Verification items for the finished model (mm, model axes). A direction names the side the tool comes from. Coordinates: 2 decimals unless noted, no trailing zeros. Loops run counter-clockwise (first coordinate to the right, second up) from the corner with the lowest first, then second, coordinate; pieces in that order, holes last. Notation, with made-up numbers: (60, 28.25) -> (93, 28.25) arc R12 cw to (93, 47.25) -> close; hole circle Ø2 at (2.25, 42). An arc over 180 degrees is marked (long way). Write item = value, one per line.
Autodesk Inventor part; units mm, degrees
ref_plane "YZ Plane" through (0, 0, 0) normal (1, 0, 0) x (0, 1, 0)
ref_plane "XZ Plane" through (0, 0, 0) normal (0, 1, 0) x (-1, 0, 0)
ref_plane "XY Plane" through (0, 0, 0) normal (0, 0, 1) x (1, 0, 0)
sketch "Szkic1" plane through (0, 0, 0) normal (0, 0, 1) x (1, 0, 0)
  line L0 (0, 0) -> (17, 0)
  line L1 (17, 0) -> (17, -2)
  line L2 (17, -2) -> (-2, -2)
  line L3 (-2, -2) -> (-2, 148)
  line L4 (-2, 148) -> (-16, 148)
  line L5 (-16, 148) -> (-16, 150)
  line L6 (-16, 150) -> (0, 150)
  line L7 (0, 150) -> (0, 0)
  line L8 (0, 150) -> (17, 150)
  line L9 (17, 150) -> (17, 0)
  line L10 (-16, 150) -> (-16, 160)
  line L11 (-16, 160) -> (-10, 160)
  line L12 (-10, 160) -> (-10, 162)
  line L13 (-10, 162) -> (-18, 162)
  line L14 (-18, 162) -> (-18, 135)
  line L15 (-18, 135) -> (-10, 135)
  line L16 (-10, 135) -> (-10, 137)
  line L17 (-10, 137) -> (-16, 137)
  line L18 (-16, 137) -> (-16, 148)
  dimension "d0" = 17
  dimension "d1" = 2
  dimension "d2" = 2
  dimension "d3" = 148
  dimension "d4" = 2
  dimension "d5" = 14
  dimension "d10" = 2
  dimension "d11" = 6
  dimension "d12" = 2
  dimension "d13" = 2
  dimension "d14" = 27
  dimension "d15" = 11
extrude "Wyciągnięcie proste1" add sketch "Szkic1" along normal blind 400 contours L0 L1 L2 L3 L4 L5 L6 L7 | L5 L18 L17 L16 L15 L14 L13 L12 L11 L10
extrude "Wyciągnięcie proste2" add sketch "Szkic1" along normal blind 2 contours L7 L8 L9 L0
sketch "Szkic2" plane through (0, 0, 400) normal (0, 0, 1) x (1, 0, 0)
  line L0 (-16, 148) -> (-2, 148)
  line L1 (-2, 148) -> (-2, -2)
  line L2 (17, 0) -> (0, 0)
  line L3 (-16, 148) -> (-2, 148)
  line L4 (-2, 148) -> (-2, 67)
  line L5 (-2, 67) -> (-16, 67)
  line L6 (-16, 67) -> (-16, 148)
  line L7 (-9, 67) -> (-9, 148) construction
  point P0 (-9, 75)
  point P1 (-9, 139)
  dimension "d16" = 75
  dimension "d17" = 64
  dimension "d18" = 8
extrude "Wyciągnięcie proste3" add sketch "Szkic2" against normal blind 2
hole "Otwór1" at (-9, 75, 400) at (-9, 139, 400) direction (0, 0, -1) diameter 4 end up to surface
properties part number "bok szuflady metalbox 150x400mm lewy"
1) Release check for a two-part mould opening along Y. For faces 1 (the face through (-2, 72, 197)), 2 (the face through (-14, 162, 197)), 3 (the face through (-16, 142, 196)) record: pulls with the +Y half, pulls with the -Y half, needs draft (parallel to the pull), parting line crosses it, or undercut.
Ans:
face_1 = needs draft
face_2 = pulls with the +Y half
face_3 = undercut
2) Sectioned sample at B-B, the plane x = 6. Record the cut outline in (y, z).
Ans:
outline = (-2, 0) -> (150, 0) -> (150, 2) -> (0, 2) -> (0, 400) -> (-2, 400) -> close
3) Sectioned sample at A-A, the plane z = 27.5. Record the cut outline in (x, y).
Ans:
outline = (-18, 135) -> (-10, 135) -> (-10, 137) -> (-16, 137) -> (-16, 148) -> (-2, 148) -> (-2, -2) -> (17, -2) -> (17, 0) -> (0, 0) -> (0, 150) -> (-16, 150) -> (-16, 160) -> (-10, 160) -> (-10, 162) -> (-18, 162) -> close
4) Material ranges on line 1 (Y direction, x = -9, z = 399.4); line 2 (X direction, y = 139, z = 399.2); line 3 (X direction, y = 75, z = 398.95), recorded low to high.
Ans:
line_1 = 67 to 73, 77 to 137, 141 to 150
line_2 = -18 to -11, -7 to 0
line_3 = -16 to -11, -7 to 0
5) Sectioned sample at D-D, the plane y = 58. Record the cut outline in (x, z).
Ans:
outline = (-2, 0) -> (17, 0) -> (17, 2) -> (0, 2) -> (0, 400) -> (-2, 400) -> close
6) Depth check by flat-ended pin: pin 1 Ø11 at (x, y) = (-8, 115) entering from -Z; pin 2 Ø4 at (x, z) = (-9, 305.5) entering from -Y; pin 3 Ø1 at (x, z) = (-12, 399.5) entering from -Y. Enter the tip coordinate at first touch or a pass-through.
Ans:
pin_1 = 398
pin_2 = 135
pin_3 = 67
7) Tool access check on faces 4 (the face through (-9, 148, 196)), 5 (the face through (-7, 99, 400)), 6 (the face through (-16, 155, 197)), 7 (the face through (8, 0, 198)), 8 (the face through (7, 81, 0)). Record the directions out of +Z, -Z, +X, -X, +Y, -Y that give a thin tool (end or side, any length) a straight path to the whole face; none if there is none.
Ans:
face_4 = -Z
face_5 = +Z, +X, -X, +Y, -Y
face_6 = +Z, -Z, +X
face_7 = +Z, +X, +Y
face_8 = -Z, +X, -X, +Y, -Y
8) Sectioned sample at C-C, the plane y = 98.5. Record the cut outline in (x, z), plus the area to 3 significant figures.
Ans:
outline = (-16, 398) -> (-2, 398) -> (-2, 0) -> (17, 0) -> (17, 2) -> (0, 2) -> (0, 400) -> (-16, 400) -> close
area = 862 mm2
